```python
from build123d import *

# Parameters (mm, degrees)
SKETCH1_W           = 7
SKETCH1_H           = 7
BOSS_EXTRUDE1_DEPTH = 3
CUT_EXTRUDE1_DEPTH  = 7
CUT_EXTRUDE2_DEPTH  = 11
SKETCH4_R           = 1.8
CUT_EXTRUDE3_DEPTH  = 0.8
CUT_EXTRUDE4_DEPTH  = 0.4


with BuildPart() as part:
    # Sketch1 → Boss-Extrude1 (new body)
    with BuildSketch(Plane(origin=(0, 0, 0), x_dir=(1, 0, 0), z_dir=(0, 1, 0))):
        with Locations((3.5, 3.5)):
            Rectangle(SKETCH1_W, SKETCH1_H)
    extrude(amount=BOSS_EXTRUDE1_DEPTH)

    # Sketch2 → Cut-Extrude1 (cut)
    with BuildSketch(Plane.XY):
        Polygon((0, 0), (0.7, 3), (0, 3), align=None)
        Polygon((7, 0), (6.3, 3), (7, 3), align=None)
    extrude(amount=-CUT_EXTRUDE1_DEPTH, mode=Mode.SUBTRACT)

    # Sketch3 → Cut-Extrude2 (cut)
    with BuildSketch(Plane(origin=(0, 0, 0), x_dir=(0, 0, -1), z_dir=(1, 0, 0))):
        Polygon((0, 0), (0.7, 3), (0, 3), align=None)
        Polygon((7, 3), (6.3, 3), (7, 0), align=None)
    extrude(amount=CUT_EXTRUDE2_DEPTH, mode=Mode.SUBTRACT)

    # Sketch4 → Cut-Extrude3 (cut)
    with BuildSketch(Plane.XZ):
        with Locations(Location((3.5, -3.5, 0), (0, 0, 270))):
            Circle(SKETCH4_R)
    extrude(amount=-CUT_EXTRUDE3_DEPTH, mode=Mode.SUBTRACT)

    # Sketch5 → Cut-Extrude4 (cut)
    with BuildSketch(Plane(origin=(0, 3, 0), x_dir=(1, 0, 0), z_dir=(0, 1, 0))):
        with BuildLine():
            Line((2.104762775, 5.272776287), (3.388516782, 5.272776287))
            add(Edge.make_bspline(
                [(3.388516782, 5.272776287), (3.423578188, 5.272794463), (3.49185089, 5.272829856), (3.590932455, 5.26871941), (3.683586456, 5.264584843), (3.769546954, 5.256308342), (3.849112172, 5.247633102), (3.922424888, 5.236649595), (3.989021979, 5.222573028), (4.031018068, 5.211471972), (4.051076878, 5.206169716)],
                knots=[0, 0, 0, 0, 1.259756885, 2.453039283, 3.563158368, 4.591894114, 5.55549294, 6.43918076, 7.254497783, 8, 8, 8, 8], degree=3))
            add(Edge.make_bspline(
                [(4.051076878, 5.206169716), (4.076161646, 5.197994199), (4.125879345, 5.181790425), (4.198767023, 5.153398715), (4.267824301, 5.118187268), (4.335613125, 5.081173488), (4.399107207, 5.037408997), (4.461666778, 4.991877903), (4.519231823, 4.939134894), (4.594720977, 4.865423065), (4.680859839, 4.762740157), (4.771103422, 4.626536439), (4.847485635, 4.477034119), (4.899673474, 4.343085246), (4.93491273, 4.229217389), (4.957948246, 4.137924241), (4.977515517, 4.041758553), (4.993580306, 3.940696082), (5.006062185, 3.834736813), (5.015355077, 3.72390899), (5.019881652, 3.608116873), (5.020906543, 3.529323002), (5.021429442, 3.489122441)],
                knots=[0, 0, 0, 0, 0.745524535, 1.477620414, 2.207090574, 2.934465325, 3.657932502, 4.384347339, 5.118673636, 5.861150177, 7.365375624, 8.894729774, 10.468936425, 12.099947606, 12.950091786, 13.83580991, 14.759228729, 15.722225242, 16.726454549, 17.773376212, 18.863978586, 20, 20, 20, 20], degree=3))
            add(Edge.make_bspline(
                [(5.021429442, 3.489122441), (5.020474912, 3.419643533), (5.01862887, 3.285272719), (4.99724236, 3.091376197), (4.966421697, 2.911281512), (4.931680416, 2.798930618), (4.914858929, 2.744531095)],
                knots=[0, 0, 0, 0, 1.103207939, 2.133582005, 3.096293362, 4, 4, 4, 4], degree=3))
            add(Edge.make_bspline(
                [(4.914858929, 2.744531095), (4.903751174, 2.713315462), (4.881900487, 2.651909444), (4.843663423, 2.56333096), (4.802348006, 2.479035433), (4.75761154, 2.399089275), (4.709228004, 2.323852087), (4.657016426, 2.253548907), (4.601786127, 2.187254174), (4.561774971, 2.146449452), (4.541862134, 2.126141671)],
                knots=[0, 0, 0, 0, 1.090884612, 2.145940218, 3.175104604, 4.181306866, 5.161203701, 6.118658341, 7.063689906, 8, 8, 8, 8], degree=3))
            add(Edge.make_bspline(
                [(4.541862134, 2.126141671), (4.509638353, 2.097162572), (4.443188324, 2.037403538), (4.326091991, 1.963449345), (4.193740208, 1.898101387), (4.098005021, 1.864533226), (4.048272391, 1.847095197)],
                knots=[0, 0, 0, 0, 0.908140292, 1.872714733, 2.8949153, 4, 4, 4, 4], degree=3))
            add(Edge.make_bspline(
                [(4.048272391, 1.847095197), (4.028252483, 1.840946487), (3.986702201, 1.828185158), (3.920820132, 1.814555795), (3.85048937, 1.800197126), (3.774898904, 1.791547242), (3.6948334, 1.782425557), (3.60965481, 1.77730424), (3.519658403, 1.773668403), (3.457932074, 1.773078068), (3.426377359, 1.772776287)],
                knots=[0, 0, 0, 0, 0.799129865, 1.658552685, 2.566799617, 3.538529252, 4.561352959, 5.643373779, 6.795284424, 8, 8, 8, 8], degree=3))
            Line((3.426377359, 1.772776287), (2.104762775, 1.772776287))
            Line((2.104762775, 1.772776287), (2.104762775, 5.272776287))
        make_face()
        with BuildLine():
            Line((2.777839698, 4.689442953), (2.777839698, 2.35610962))
            Line((2.777839698, 2.35610962), (3.331725916, 2.35610962))
            add(Edge.make_bspline(
                [(3.331725916, 2.35610962), (3.356732427, 2.356307939), (3.404879513, 2.356689778), (3.474549579, 2.357811767), (3.538575784, 2.360849202), (3.597293536, 2.36399549), (3.65054997, 2.369193709), (3.698576813, 2.374306355), (3.741106724, 2.38145884), (3.767374243, 2.387104916), (3.779742743, 2.389763466)],
                knots=[0, 0, 0, 0, 1.333384787, 2.567275092, 3.714769766, 4.750907381, 5.701951617, 6.567520054, 7.325492842, 8, 8, 8, 8], degree=3))
            add(Edge.make_bspline(
                [(3.779742743, 2.389763466), (3.808711174, 2.397493681), (3.865134036, 2.412550099), (3.944357438, 2.44611519), (4.01604441, 2.486607799), (4.08139549, 2.535298421), (4.140290341, 2.596832105), (4.190564295, 2.675528863), (4.237091515, 2.769385848), (4.268953366, 2.859230456), (4.291823741, 2.939477558), (4.307305109, 3.006830931), (4.319539616, 3.07970047), (4.330062887, 3.157798585), (4.338565941, 3.241024846), (4.343856943, 3.329679796), (4.347468084, 3.423654914), (4.348052123, 3.488183941), (4.348352519, 3.521374043)],
                knots=[0, 0, 0, 0, 1.038686998, 2.023088296, 2.974059649, 3.888265163, 4.839857954, 5.909819677, 7.113156087, 8.466843969, 9.20827164, 10.006482943, 10.861893492, 11.769681931, 12.739021491, 13.762258324, 14.849031541, 16, 16, 16, 16], degree=3))
            add(Edge.make_bspline(
                [(4.348352519, 3.521374043), (4.348054433, 3.554564247), (4.347476984, 3.618859926), (4.34387138, 3.712134321), (4.338610098, 3.799393203), (4.330046489, 3.880744437), (4.319686346, 3.956300457), (4.307308533, 4.0261252), (4.291920489, 4.089760429), (4.26903066, 4.165360255), (4.234330859, 4.250336809), (4.187111202, 4.343245577), (4.129123838, 4.422434336), (4.065053447, 4.491226906), (3.991179205, 4.547839715), (3.909400596, 4.595256239), (3.817937068, 4.632059083), (3.752876188, 4.647734621), (3.719446269, 4.655789107)],
                knots=[0, 0, 0, 0, 1.117996097, 2.165769068, 3.143980016, 4.062055362, 4.920439205, 5.712587309, 6.449616741, 7.124491204, 8.371470382, 9.537068822, 10.625202851, 11.666538334, 12.693249444, 13.747832046, 14.842779399, 16, 16, 16, 16], degree=3))
            add(Edge.make_bspline(
                [(3.719446269, 4.655789107), (3.704976171, 4.658477854), (3.673118556, 4.664397445), (3.620253908, 4.671311562), (3.558231897, 4.676442427), (3.486736347, 4.68168059), (3.406056748, 4.684670369), (3.31585552, 4.687790688), (3.21651011, 4.688856584), (3.147096928, 4.68924188), (3.110872551, 4.689442953)],
                knots=[0, 0, 0, 0, 0.578738571, 1.274160813, 2.095454135, 3.025967819, 4.093109015, 5.270126069, 6.575371698, 8, 8, 8, 8], degree=3))
            Line((3.110872551, 4.689442953), (2.777839698, 4.689442953))
        make_face(mode=Mode.SUBTRACT)
    extrude(amount=-CUT_EXTRUDE4_DEPTH, mode=Mode.SUBTRACT)


solid = part.part
```
Can you work these out from the model? Positions are in its coordinate system, mm. A direction names the side the tool comes from. Give positions to 0.01 mm unless a question says otherwise; leave off trailing zeros. Order: outer loops, then holes, each group sorted by start corner. A loop starts at its lowest first (then second) coordinate and runs counter-clockwise, first axis right, second up. Notation, with made-up numbers: M 64.5,49.25 L 73.5,49.25 A9 cw 73.5,62.25 Z; hole C -34,-27 d11. An arc over 180 degrees is marked long. Write item = value, one per line. Start each with the question number.
Q1. Suppose I cut it at B-B (x = 2.5). Write out the boundary of the cut face in (y, z).
Q2. Will this pin go through, and if not, where does the flat tip stop? pin 1 Ø1 at (y, z) = (1.5, -1) entering from -X.
Q3. I need wall thicknesses on probe 1 along X at (y, z) = (2.8, -3.5); probe 2 along X at (y, z) = (2.8, -4.5); probe 3 along Z at (x, y) = (4.5, 0.7). Which ranges of each line are inside material? Lowest first, please. Write a range as [from, to].
Q4. Suppose I cut it at C-C (z = -5.5). Write out the boundary of the cut face in (x, y), plus the area to 3 significant figures.
Q5. We'd pull the mould along Z, two halves only. Please class faces 4 (the flat face through (0.345, 1.479, -3.451)), 5 (the flat face through (3.451, 1.479, -0.345)), 6 (the cylindrical face through (4.041, 0.394, -5.217)): pulls with the +Z half, pulls with the -Z half, needs draft (parallel to the pull), parting line crosses it, or undercut.
Q6. Suppose I cut it at A-A (y = 2.1). Write out the boundary of the cut face in (x, z), plus the area to 3 significant figures.
Q7. For faces 1 (the flat face through (4, 0.8, -3)), 2 (the flat face through (2.6, 2.6, -3.5)), 3 (the flat face through (3.451, 1.521, -6.645)), which set-ups out of +Z, -Z, +X, -X, +Y, -Y let a thin tool reach every point of the face, with its end or its side?
Check result:
q1.outline = M 0,-7 L 3,-6.3 L 3,-5.27 L 2.6,-5.27 L 2.6,-1.77 L 3,-1.77 L 3,-0.7 L 0,0 L 0,-2 L 0.8,-2 L 0.8,-5 L 0,-5 Z
q2.pin_1 = 0.23
q3.probe_1 = [0.65, 2.1], [2.78, 4.35], [5.02, 6.35]
q3.probe_2 = [0.65, 2.1], [2.78, 4.05], [4.83, 6.35]
q3.probe_3 = [-6.84, -5], [-2, -0.16]
q4.outline = M 0,0 L 7,0 L 6.3,3 L 0.7,3 Z
q4.area = 18.9 mm2
q5.face_4 = needs draft
q5.face_5 = pulls with the +Z half
q5.face_6 = undercut
q6.outline = M 0.49,-6.51 L 6.51,-6.51 L 6.51,-0.49 L 0.49,-0.49 Z
q6.area = 36.2 mm2
q7.face_1 = -Y
q7.face_2 = +Y
q7.face_3 = -Z, +X, -X, +Y
